Model file for the job. Use its own axes, mm. A direction names the side the tool comes from. Coordinates: 2 decimals unless noted, no trailing zeros. Loops run counter-clockwise (first coordinate to the right, second up) from the corner with the lowest first, then second, coordinate; pieces in that order, holes last.
from build123d import *

# Parameters (mm, degrees)
SKETCH1_R           = 1.65
BOSS_EXTRUDE1_DEPTH = 3


with BuildPart() as part:
    # Sketch1 → Boss-Extrude1 (new body)
    with BuildSketch(Plane(origin=(0, 0, 0), x_dir=(1, 0, 0), z_dir=(0, 1, 0))):
        Polygon((-40, -1), (-34, 9), (34, 9), (40, -1), (40, -6), (24, -6), (24, -9), (8, -9), (8, -6), (-8, -6), (-8, -9), (-24, -9), (-24, -6), (-40, -6), align=None)
        with Locations((-20, 3.003103662)):
            Circle(SKETCH1_R, mode=Mode.SUBTRACT)
        with Locations((20, 3.003103662)):
            Circle(SKETCH1_R, mode=Mode.SUBTRACT)
    extrude(amount=BOSS_EXTRUDE1_DEPTH)


solid = part.part
Q1. Slice it at D-D (y = 2.2). List the corners of the cut face in (x, z), and give its area (3 significant figures).
Answers:
outline: (-40, 1) - (-34, -9) - (34, -9) - (40, 1) - (40, 6) - (24, 6) - (24, 9) - (8, 9) - (8, 6) - (-8, 6) - (-8, 9) - (-24, 9) - (-24, 6) - (-40, 6) - close; hole circle Ø3.3 at (-20, -3); hole circle Ø3.3 at (20, -3)
area: 1,220 mm2
Q2. Slice it at A-A (x = 20). List the corners of the cut face in (y, z), and give its area (3 significant figures).
Answers:
outline: (0, -9) - (3, -9) - (3, -4.65) - (0, -4.65) - close; (0, -1.35) - (3, -1.35) - (3, 9) - (0, 9) - close
area: 44.1 mm2
Q3. Slice it at B-B (z = 7.75). List the corners of the cut face in (x, y).
Answers:
outline: (-24, 0) - (-8, 0) - (-8, 3) - (-24, 3) - close; (8, 0) - (24, 0) - (24, 3) - (8, 3) - close
Q4. Which spindle directions (+Z, -Z, +X, -X, +Y, -Y) get a long thin tool onto all of the face, cutting with end or side? Do faces 5 (the flat face through (-24, 1, 8)), 6 (the flat face through (0, 1, 6)), 7 (the flat face through (1, 3, 0)), 8 (the flat face through (24, 1, 7)). Say none if no direction does.
Answers:
face 5: +Z, -X, +Y, -Y
face 6: +Z, +Y, -Y
face 7: +Z, -Z, +X, -X, +Y
face 8: +Z, +X, +Y, -Y
Q5. Flat gauge pins, fed straight in: P1, Ø1.5, axis at x = -1.5, y = 1, coming from the +Z side; P2, Ø0.9, axis at y = 1.5, z = 7.5, coming from the +X side; P3, Ø4, axis at x = 1.5, z = -0.5, coming from the -Y side; P4, Ø0.9, axis at y = 1, z = 7.5, coming from the -X side. Where does each tip first touch, or does it go through?
Answers:
P1: stops at z = 6
P2: stops at x = 24
P3: stops at y = 0
P4: stops at x = -24
Q6. Mould opens along Z. For faces 1 (the flat face through (16, 1, 9)), 2 (the cylindrical face through (18.784, 1.479, -4.118)), 3 (the cylindrical face through (-21.216, 1.479, -4.118)), 4 (the flat face through (-8, 1, 7)) say: +Z half, -Z half, draft (parallel to the pull), parting line (faces both ways), or undercut.
Answers:
face 1: +Z half
face 2: undercut
face 3: undercut
face 4: draft
Q7. Slice it at C-C (z = -3.75). List the corners of the cut face in (x, y).
Answers:
outline: (-37.15, 0) - (-21.47, 0) - (-21.47, 3) - (-37.15, 3) - close; (-18.53, 0) - (18.53, 0) - (18.53, 3) - (-18.53, 3) - close; (21.47, 0) - (37.15, 0) - (37.15, 3) - (21.47, 3) - close
Q8. Drill centre lines: line 1 (X direction, y = 2.4, z = -1.5); line 2 (X direction, y = 1.65, z = -4.5); line 3 (Z direction, x = -29.5, y = 0.8). Where is each one in solid material? Low to high.
Answers:
line 1: x = -38.5 to -20.68, -19.32 to 19.32, 20.68 to 38.5
line 2: x = -36.7 to -20.69, -19.31 to 19.31, 20.69 to 36.7
line 3: z = -9 to 6
